Check sheet for the drawn part. Datum: minimum x, y, z corner. Units: mm. A direction names the side the tool comes from. Give positions to 0.01 mm unless a question says otherwise; leave off trailing zeros. Write each loop counter-clockwise with the first axis right and the second up, starting at its lowest first coordinate (ties: lowest second). Pieces come first, ordered by that corner, then holes. Notation, with made-up numbers: (-32, 39.5) -> (24, 39.5) arc R24 cw to (24, 78.5) -> close; hole circle Ø4 at (34, 38). An arc over 180 degrees is marked (long way). Write item = value, one per line. Start each with the question number.
1. Depth check by flat-ended pin: P1, Ø4, axis at y = 19, z = 115, coming from the -X side (1 decimal); P2, Ø10, axis at x = 27.5, z = 136, coming from the +Y side; P3, Ø1.5, axis at x = 36.5, y = 6, coming from the -Z side. Enter the tip coordinate at first touch or a pass-through.
2. Thickness scan on line 1 along Y through (x, z) = (34, 70); line 2 along Z through (x, y) = (3, 39) (1 decimal); line 3 along Y through (x, z) = (3.25, 15). Record the ranges inside material, lowest first.
3. Cross-section at A-A, the plane z = 170. Record the cut outline in (x, y).
4. Cross-section at C-C, the plane y = 3. Record the cut outline in (x, z).
5. Cross-section at D-D, the plane z = 54.5. Record the cut outline in (x, y).
6. Set-up check for the marked faces 1, 2 and 3: record each of +Z, -Z, +X, -X, +Y, -Y from which the full face is reachable in a straight line by a thin tool's end or side.
7. Cross-section at B-B, the plane y = 13.5. Record the cut outline in (x, z).
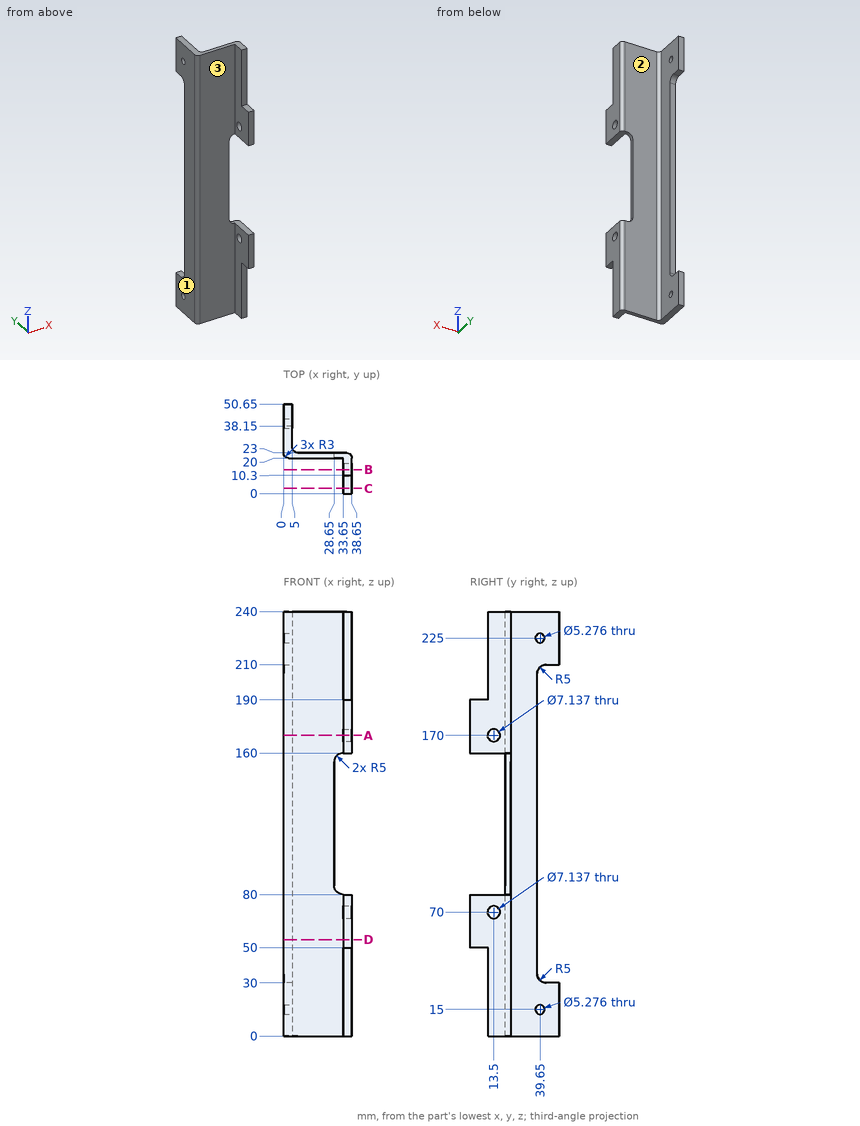
Answers:
q1.P1 = 0.8
q1.P2 = 23
q1.P3 = 50
q2.line_1 = 0 to 9.93, 17.07 to 23
q2.line_2 = 0 to 12.4, 17.6 to 32.2, 207.8 to 222.4, 227.6 to 240
q2.line_3 = 20 to 37.01, 42.29 to 50.65
q3.outline = (0, 23) arc R3 ccw to (3, 20) -> (33.65, 20) -> (33.65, 17.07) -> (38.65, 17.07) -> (38.65, 20) arc R3 ccw to (35.65, 23) -> (8, 23) arc R3 cw to (5, 26) -> (5, 38.15) -> (0, 38.15) -> close; (33.65, 0) -> (38.65, 0) -> (38.65, 9.93) -> (33.65, 9.93) -> close
q4.outline = (33.65, 50) -> (38.65, 50) -> (38.65, 80) -> (33.65, 80) -> close; (33.65, 160) -> (38.65, 160) -> (38.65, 190) -> (33.65, 190) -> close
q5.outline = (0, 23) arc R3 ccw to (3, 20) -> (33.65, 20) -> (33.65, 0) -> (38.65, 0) -> (38.65, 20) arc R3 ccw to (35.65, 23) -> (8, 23) arc R3 cw to (5, 26) -> (5, 38.15) -> (0, 38.15) -> close
q6.face_1 = +Z, -Z, -X, +Y, -Y
q6.face_2 = +Z, -Z, +X, +Y
q6.face_3 = +Z, -Z, -X, -Y
q7.outline = (33.65, 0) -> (38.65, 0) -> (38.65, 66.43) -> (33.65, 66.43) -> close; (33.65, 73.57) -> (38.65, 73.57) -> (38.65, 80) -> (33.65, 80) -> close; (33.65, 160) -> (38.65, 160) -> (38.65, 166.43) -> (33.65, 166.43) -> close; (33.65, 173.57) -> (38.65, 173.57) -> (38.65, 240) -> (33.65, 240) -> close
